Autodesk Inventor part; units mm, degrees
ref_plane "YZ Plane" through (0, 0, 0) normal (1, 0, 0) x (0, 1, 0)
ref_plane "XZ Plane" through (0, 0, 0) normal (0, 1, 0) x (-1, 0, 0)
ref_plane "XY Plane" through (0, 0, 0) normal (0, 0, 1) x (1, 0, 0)
sketch "Sketch1" plane through (0, 0, 0) normal (0, 0, 1) x (1, 0, 0)
  line L0 (0, 0) -> (25, 0)
  line L1 (25, 0) -> (25, 40)
  line L2 (25, 40) -> (0, 40)
  line L3 (0, 40) -> (0, 0)
  dimension "d1" = 25
  dimension "d2" = 40
  dimension "d3" = 25
extrude "Extrusion1" add sketch "Sketch1" against normal blind 30
sketch "Sketch2" plane through (25, 0, 0) normal (1, 0, 0) x (0, 0, -1)
  line L0 (0, 0) -> (30, 0)
  circle A0 centre (15, 6.56) radius 2.46
extrude "Extrusion2" cut sketch "Sketch2" against normal blind 30
sketch "Sketch3" plane through (0, 0, 0) normal (-1, 0, 0) x (0, 0, 1)
  line L0 (0, 0) -> (-30, 0)
  line L1 (-25.05, 0) -> (-4.95, 0)
  line L2 (-4.95, 0) -> (-4.95, 33.12)
  line L3 (-4.95, 33.12) -> (-25.05, 33.12)
  line L4 (-25.05, 33.12) -> (-25.05, 0)
  dimension "d11" = 20.1
extrude "Extrusion3" cut sketch "Sketch3" against normal blind 20
sketch "Sketch4" plane through (0, 0, 0) normal (0, -1, 0) x (1, 0, 0)
  line L0 (20, -4.95) -> (20, -25.05)
  line L1 (20, -15) -> (25, -15)
  line L2 (25, 0) -> (25, -30)
  line L3 (20, -8.025) -> (25, -8.025)
  line L4 (25, -8.025) -> (25, -21.975)
  line L5 (25, -21.975) -> (20, -21.975)
  line L6 (20, -21.975) -> (20, -8.025)
  line L7 (20, -8.025) -> (25, -21.975) construction
  line L8 (25, -8.025) -> (20, -21.975) construction
  line L9 (25, -12.54) -> (25, -17.46)
  point P0 (0, 0)
  point P1 (22.5, -15)
  dimension "d14" = 13.95
extrude "Extrusion4" add sketch "Sketch4" along normal blind 15
sketch "Sketch5" plane through (20, 0, 0) normal (-1, 0, 0) x (0, 0, 1)
  circle A0 centre (-15, 6.56) radius 2.46
  circle A1 centre (-15, 6.56) radius 4.7025
  circle A2 centre (-15, 6.56) radius 2.46
  circle A3 centre (-15, 6.56) radius 2.46
  point P0 (0, 0)
  dimension "d17" = 9.405
extrude "Extrusion5" cut sketch "Sketch5" against normal blind 2.1
sketch "Sketch6" plane through (25, 0, 0) normal (1, 0, 0) x (0, 0, -1)
  circle A0 centre (15, 6.56) radius 4.7025
  line L0 (15, 6.56) -> (15, 23.56)
  circle A1 centre (15, 23.56) radius 2.46
  point P0 (0, 0)
  dimension "d20" = 17
  dimension "d21" = 4.92
extrude "Extrusion6" cut sketch "Sketch6" against normal blind 10 contours A1
sketch "Sketch7" plane through (20, 0, 0) normal (-1, 0, 0) x (0, 0, 1)
  circle A0 centre (-15, 23.56) radius 2.46
  circle A1 centre (-15, 23.56) radius 4.7025
  point P0 (0, 0)
  dimension "d24" = 9.405
extrude "Extrusion7" cut sketch "Sketch7" against normal blind 2.1
sketch "Sketch9" plane through (25, 0, 0) normal (1, 0, 0) x (0, 0, -1)
  circle A0 centre (15, 6.56) radius 2.46
  circle A1 centre (15, 6.56) radius 2.46
  circle A2 centre (15, 23.56) radius 2.46
  circle A3 centre (15, 23.56) radius 2.46
  line L0 (30, 40) -> (30, 0)
  line L1 (30, 0) -> (30, 40)
  line L2 (30, 40) -> (0, 40)
  line L3 (0, 40) -> (0, 0)
  line L4 (0, 0) -> (8.025, 0)
  line L5 (21.975, 0) -> (21.975, -15)
  line L6 (21.975, -15) -> (8.025, -15)
  line L7 (8.025, -15) -> (8.025, 0)
  line L8 (0, 0) -> (8.025, 0)
  line L9 (21.975, 0) -> (30, 0)
extrude "Extrusion8" add sketch "Sketch9" along normal blind 5
sketch "Sketch10" plane through (0, 40, 0) normal (0, 1, 0) x (1, 0, 0)
  line L0 (0, 30) -> (30, 30)
  line L1 (30, 0) -> (0, 0)
  line L2 (0, 30) -> (30, 30)
  line L3 (30, 30) -> (30, 0)
  line L4 (30, 0) -> (0, 0)
  line L5 (0, 0) -> (0, 30)
extrude "Extrusion9" add sketch "Sketch10" along normal blind 30
sketch "Sketch12" plane through (30, 0, 0) normal (1, 0, 0) x (0, 0, -1)
  circle A0 centre (15, 6.56) radius 2.46
  line L0 (15, 6.56) -> (15, 15.06)
  circle A1 centre (15, 15.06) radius 2.525
  point P0 (0, 0)
  dimension "d31" = 8.5
  dimension "d33" = 5.05
extrude "Extrusion10" cut sketch "Sketch12" against normal blind 30 contours A1
sketch "Sketch14" plane through (0, 0, 0) normal (0, 0, 1) x (1, 0, 0)
  line L0 (30, 70) -> (0, 70)
  line L1 (0, 70) -> (0, 85)
  line L2 (30, 100) -> (15, 115)
  line L3 (-12, 115) -> (15, 115)
  line L4 (30, 0) -> (30, 70)
  line L5 (30, 100) -> (30, 70)
  line L6 (-9.5, 113.5) -> (-12, 115)
  line L7 (-9.5, 101.5) -> (-12, 100)
  line L8 (-7, 107.5) -> (-9.5, 101.5)
  line L9 (-7, 107.5) -> (-9.5, 113.5)
  line L10 (0, 100) -> (0, 85)
  line L11 (0, 100) -> (-12, 100)
  point P0 (0, 0)
  dimension "d49" = 15
  dimension "d61" = 12
extrude "Extrusion12" add sketch "Sketch14" against normal blind 30
sketch "Sketch15" plane through (0, 0, -25.05) normal (-1, 0, 0) x (0, 0, 1)
  line L0 (0, 33.12) -> (20.1, 33.12)
  line L1 (20.1, 33.12) -> (20.1, 0)
  line L2 (0, 33.12) -> (20.1, 33.12)
  line L3 (20.1, 33.12) -> (20.1, 31.1)
  line L4 (20.1, 31.1) -> (0, 31.1)
  line L5 (0, 31.1) -> (0, 33.12)
  point P0 (25.05, 0)
  dimension "d57" = 2.02
extrude "Extrusion13" add sketch "Sketch15" against normal blind 20
properties part number "10mm_x_30mm"
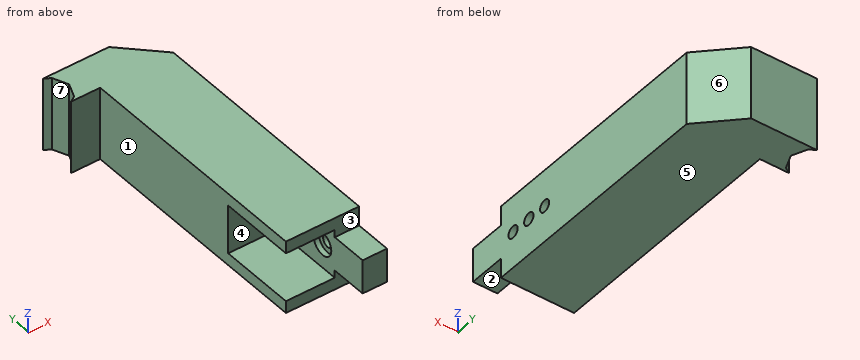
Design review of the part built by this model. Coordinates are the model's own, in mm. Face numbers are marked on the shaded views. A direction names the side the tool comes from. Give positions to 0.01 mm unless a question says otherwise; leave off trailing zeros. Order: outer loops, then holes, each group sorted by start corner. A loop starts at its lowest first (then second) coordinate and runs counter-clockwise, first axis right, second up. Notation, with made-up numbers: (75.25, 39.5) -> (81.25, 39.5) arc R35 cw to (81.25, 74.5) -> close; hole circle Ø4 at (79, 12.5). An arc over 180 degrees is marked (long way). Write each question's results on one line, items separated by ' | '. Start each with the question number.
Q1. Wall thickness on L1, parallel to Z at x = 14, y = 27; L2, parallel to Y at x = 25.25, z = -15 (3 decimals); L3, parallel to Y at x = 27.25, z = -15 (3 decimals): over which ranges is each line inside the solid? List them lowest first. Write a range as from..to.
Q2. Machinability: for the marked faces 1, 2, 3 and 4, which of the approach directions +Z, -Z, +X, -X, +Y, -Y give a long, thin tool a straight path to every point of the face, cutting with its end or side? Answer none if there is none.
Q3. Add section B-B on y = 23.56. Give the boundary of the cut face in (x, z), and give its area (3 significant figures).
Q4. Add section A-A on z = -15. State how many separate pieces and enclosed holes the cut face has, and give its area (3 significant figures).
Q5. Add section C-C on x = 18. Give the boundary of the cut face in (y, z), and give its area (3 significant figures).
Q6. Mouldability with a two-part tool opening along Y and no side actions: class the marked faces 5, 6 and 7 as +Y half, -Y half, draft (parallel to the pull), parting line (faces both ways), or undercut.
Q7. For pin 1 (5 mm diameter, centred on x = -7.5, z = -7, fed in from -Y); pin 2 (8 mm diameter, centred on x = 1.5, z = -24, fed in from -Y); pin 3 (8.5 mm diameter, centred on y = 23.56, z = -15, fed in from -X), all flat-tipped, find the tip position at first contact; note any pin that passes through.
Q8. Add section D-D on z = -26.5. Give the boundary of the cut face in (x, y), and give its area (3 significant figures).
Found:
1) L1: z = -30..-25.05, -4.95..0 | L2: y = -15..4.1, 9.02..12.535, 17.585..21.1, 26.02..104.75 | L3: y = -15..4.1, 9.02..12.535, 17.585..21.1, 26.02..102.75
2) face 1: +Z, -Z, -X, -Y | face 2: -Z, +X, -X, -Y | face 3: +Z, +X, -X, -Y | face 4: -X, -Y
3) outline: (0, -30) -> (30, -30) -> (30, -17.46) -> (22.1, -17.46) -> (22.1, -19.7) -> (20, -19.7) -> (20, -25.05) -> (0, -25.05) -> close; (0, -4.95) -> (20, -4.95) -> (20, -10.3) -> (22.1, -10.3) -> (22.1, -12.54) -> (30, -12.54) -> (30, 0) -> (0, 0) -> close | area: 439 mm2
4) separate pieces: 4 | enclosed holes: 0 | area: 2,830 mm2
5) outline: (0, -30) -> (112, -30) -> (112, 0) -> (0, 0) -> (0, -4.95) -> (31.1, -4.95) -> (31.1, -25.05) -> (0, -25.05) -> close | area: 2,730 mm2
6) face 5: draft | face 6: +Y half | face 7: undercut
7) pin 1: stops at y = 100 | pin 2: stops at y = 0 | pin 3: stops at x = 22.1
8) outline: (-12, 100) -> (0, 100) -> (0, 0) -> (30, 0) -> (30, 100) -> (15, 115) -> (-12, 115) -> (-9.5, 113.5) -> (-7, 107.5) -> (-9.5, 101.5) -> close | area: 3,470 mm2
